```python
from build123d import *

# Parameters (mm, degrees)
SKETCH1_R           = 10.9
SKETCH1_R_2         = 6.75
BOSS_EXTRUDE1_DEPTH = 1


with BuildPart() as part:
    # Sketch1 → Boss-Extrude1 (new body)
    with BuildSketch(Plane.XY):
        with BuildLine():
            Line((-15, 20), (15, 20))
            Line((15, 20), (29.736161147, 14.636475975))
            ThreePointArc((29.736161147, 14.636475975), (33.553216354, 11.7075465), (35, 7.118935009))
            Line((35, 7.118935009), (35, -7.118935009))
            ThreePointArc((35, -7.118935009), (33.553216354, -11.7075465), (29.736161147, -14.636475975))
            Line((29.736161147, -14.636475975), (15, -20))
            Line((15, -20), (-15, -20))
            Line((-15, -20), (-29.736161147, -14.636475975))
            ThreePointArc((-29.736161147, -14.636475975), (-33.553216354, -11.7075465), (-35, -7.118935009))
            Line((-35, -7.118935009), (-35, 7.118935009))
            ThreePointArc((-35, 7.118935009), (-33.553216354, 11.7075465), (-29.736161147, 14.636475975))
            Line((-29.736161147, 14.636475975), (-15, 20))
        make_face()
        Circle(SKETCH1_R, mode=Mode.SUBTRACT)
        with Locations((24, 0)):
            Circle(SKETCH1_R_2, mode=Mode.SUBTRACT)
        with Locations(Location((-24, 0, 0), (0, 0, 180))):
            Circle(SKETCH1_R_2, mode=Mode.SUBTRACT)
    extrude(amount=-BOSS_EXTRUDE1_DEPTH)


solid = part.part
```
Source: CAD feature listing. Evaluate the final solid. Frame: model axes, mm. Coordinates: 2 decimals unless noted, no trailing zeros. Order: outer loops, then holes, each group sorted by start corner. A loop starts at its lowest first (then second) coordinate and runs counter-clockwise, first axis right, second up. Notation, with made-up numbers: M -19,72 L 7,72 A22 ccw 7,99 Z; hole C -14.75,21 d4. An arc over 180 degrees is marked long. Write each question's results on one line, items separated by ' | '. Start each with the question number.
1) Contact query for a flat-ended pin moving along its axis: pin 1 Ø1.5 at (x, y) = (3.5, -12.5) entering from +Z. Output: stop coordinate, or through.
2) Line query: line 1 (Y direction, x = 0, z = -0.45); line 2 (Y direction, x = -24, z = -0.4); line 3 (X direction, y = 5, z = -0.9). Output: solid intervals per line, ascending. Write a range as from..to.
3) Section query D-D (y = -4). Return the cut outline in (x, z), plus the area to 3 significant figures.
4) Section query A-A (y = 0). Return the cut outline in (x, z).
5) Section query C-C (z = -0.8). Return the cut outline in (x, y), plus the area to 3 significant figures.
6) Draft query along Y for faces 1 (the face through (10.4, 3.27, -0.49)), 2 (the face through (8, 9, -1)), 3 (the face through (-33.592, 11.651, -0.493)). Return one class per face: released by +Y, released by -Y, zero draft, split by the parting line, or undercut.
7) Section query B-B (x = 8.5). Return the cut outline in (y, z), plus the area to 3 significant figures.
Answers:
1) pin 1: stops at z = 0
2) line 1: y = -20..-10.9, 10.9..20 | line 2: y = -16.72..-6.75, 6.75..16.72 | line 3: x = -35..-28.53, -19.47..-9.69, 9.69..19.47, 28.53..35
3) outline: M -35,-1 L -29.44,-1 L -29.44,0 L -35,0 Z; M -18.56,-1 L -10.14,-1 L -10.14,0 L -18.56,0 Z; M 10.14,-1 L 18.56,-1 L 18.56,0 L 10.14,0 Z; M 29.44,-1 L 35,-1 L 35,0 L 29.44,0 Z | area: 28.0 mm^2
4) outline: M -35,-1 L -30.75,-1 L -30.75,0 L -35,0 Z; M -17.25,-1 L -10.9,-1 L -10.9,0 L -17.25,0 Z; M 10.9,-1 L 17.25,-1 L 17.25,0 L 10.9,0 Z; M 30.75,-1 L 35,-1 L 35,0 L 30.75,0 Z
5) outline: M -35,-7.12 A8 ccw -29.74,-14.64 L -15,-20 L 15,-20 L 29.74,-14.64 A8 ccw 35,-7.12 L 35,7.12 A8 ccw 29.74,14.64 L 15,20 L -15,20 L -29.74,14.64 A8 ccw -35,7.12 Z; hole C -24,0 d13.5; hole C 0,0 d21.8; hole C 24,0 d13.5 | area: 1,830 mm^2
6) face 1: undercut | face 2: zero draft | face 3: released by +Y
7) outline: M -20,-1 L -6.82,-1 L -6.82,0 L -20,0 Z; M 6.82,-1 L 20,-1 L 20,0 L 6.82,0 Z | area: 26.4 mm^2
